The model under review builds one solid part; all positions refer to its coordinate system, in mm. A direction names the side the tool comes from. Coordinates: 2 decimals unless noted, no trailing zeros. Order: outer loops, then holes, each group sorted by start corner. A loop starts at its lowest first (then second) coordinate and runs counter-clockwise, first axis right, second up. Notation, with made-up numbers: M 71.25,16 L 119.25,16 A19 cw 119.25,39 Z; hole C -23.75,7.5 d3. An arc over 180 degrees is marked long. Answer as CSV lines item,"result". Start each with the question number.
Q1. Machinability: for faces 1 (the face through (-5, 47, 25)), 2 (the face through (5, 47, 25)), 3 (the face through (0, 47, 29.365)), which of the approach directions +Z, -Z, +X, -X, +Y, -Y give a long, thin tool a straight path to every point of the face, cutting with its end or side? Answer none if there is none.
Q2. Consider section A-A on x = 0. Write out the cut boundary in (y, z).
Q3. Consider section C-C on y = 78.5. Write out the cut boundary in (x, z), and give its area (3 significant figures).
Q4. Wall thickness on L1, parallel to Y at x = 3, z = 23.5; L2, parallel to Z at x = 0, y = 66.5; L3, parallel to X at y = 74.5, z = 21: over which ranges is each line inside the solid? List them lowest first. Write a range as [from, to].
Q5. Consider section D-D on x = -16. Write out the cut boundary in (y, z), and give its area (3 significant figures).
Q6. Consider section B-B on z = 11.5. Write out the cut boundary in (x, y), and give its area (3 significant figures).
Q7. For P1, Ø4.5, axis at y = 58.5, z = 24, coming from the +X side; P2, Ø5, axis at x = -4.5, y = 143.5, coming from the -Z side; P3, Ø11.5, axis at x = 1, z = 26.5, coming from the -Y side, all flat-tipped, find the tip position at first contact; note any pin that passes through.
from build123d import *

# Parameters (mm, degrees)
F0_R      = 20
F1_DEPTH  = 20
F1_FACE_R = 20
F3_DEPTH  = 55
F4_R      = 20
F5_DEPTH  = 125


with BuildPart() as f1:
    # F0 (on Front) → F1 (new body)
    with BuildSketch(Plane.XZ):
        Circle(F0_R)
    extrude(amount=-F1_DEPTH)

    # F2 (on face) + F1_face (on face) → F3 (join)
    with BuildSketch(Plane(origin=(0, 20, 0), x_dir=(-1, 0, 0), z_dir=(0, 1, 0))):
        with BuildLine():
            ThreePointArc((6.363636, 18.960594), (0, 20), (-6.363636, 18.960594))
            ThreePointArc((-6.363636, 18.960594), (-11.677484, -16.236883), (20, 0))
            ThreePointArc((20, 0), (16.236883, 11.677484), (6.363636, 18.960594))
        make_face()
        with BuildLine():
            ThreePointArc((-5, 20.856654), (-5.376312, 19.688905), (-6.363636, 18.960594))
            ThreePointArc((-6.363636, 18.960594), (0, 20), (6.363636, 18.960594))
            ThreePointArc((6.363636, 18.960594), (5.376312, 19.688905), (5, 20.856654))
            Line((5, 20.856654), (5, 29.364917))
            Line((5, 29.364917), (-5, 29.364917))
            Line((-5, 29.364917), (-5, 20.856654))
        make_face()
    with BuildSketch(Plane(origin=(0, 20, 0), x_dir=(1, 0, 0), z_dir=(0, 1, 0))):
        Circle(F1_FACE_R)
    extrude(amount=F3_DEPTH)

    # F4 (on face) → F5 (join)
    with BuildSketch(Plane(origin=(0, 75, 0), x_dir=(-1, 0, 0), z_dir=(0, 1, 0))):
        Circle(F4_R)
    extrude(amount=F5_DEPTH)


solid = f1.part
Evaluation:
1,face 1,"+Z, -X, +Y, -Y"
1,face 2,"+Z, +X, +Y, -Y"
1,face 3,"+Z, +X, -X, +Y, -Y"
2,outline,"M 0,-20 L 200,-20 L 200,20 L 75,20 L 75,29.36 L 20,29.36 L 20,20 L 0,20 Z"
3,outline,"C 0,0 d40"
3,area,"1,260 mm²"
4,L1,"y = [20, 75]"
4,L2,"z = [-20, 29.36]"
4,L3,"x = [-5, 5]"
5,outline,"M 0,-12 L 200,-12 L 200,12 L 0,12 Z"
5,area,"4,800 mm²"
6,outline,"M -16.36,0 L 16.36,0 L 16.36,200 L -16.36,200 Z"
6,area,"6,550 mm²"
7,P1,"stops at x = 5"
7,P2,"stops at z = -19.9"
7,P3,"stops at y = 20"
